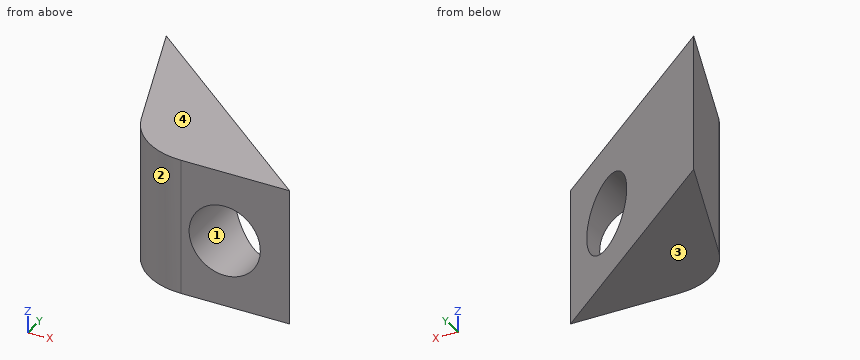
from build123d import *

# Parameters (mm, degrees)
BOSS_EXTRUDE1_DEPTH = 10
FILLET1_R           = 5
SKETCH4_R           = 2.6
CUT_EXTRUDE1_DEPTH  = 10


with BuildPart() as part:
    # Sketch2 → Boss-Extrude1 (new body)
    with BuildSketch(Plane.XY):
        Polygon((0, 0), (11.45, 0), (-4.62309301, 13.05), align=None)
    extrude(amount=BOSS_EXTRUDE1_DEPTH)

    # Fillet1
    fillet1_edges = [part.edges().sort_by_distance(p)[0] for p in [
        (0, 0, 5),
    ]]
    fillet(fillet1_edges, radius=FILLET1_R)

    # Sketch4 → Cut-Extrude1 (cut)
    with BuildSketch(Plane.XZ):
        with Locations(Location((6.713179585, 4.87, 0), (0, 0, 270))):
            Circle(SKETCH4_R)
    extrude(amount=-CUT_EXTRUDE1_DEPTH, mode=Mode.SUBTRACT)


solid = part.part
Geometry: final body of the model. Coordinates: model frame, mm. Face numbers are marked on the shaded views. Coordinates: 2 decimals unless noted, no trailing zeros. Loops run counter-clockwise (first coordinate to the right, second up) from the corner with the lowest first, then second, coordinate; pieces in that order, holes last. Notation, with made-up numbers: M 19.5,16.5 L 75.5,16.5 A23 cw 75.5,31.5 Z; hole C 26.5,73.5 d10. An arc over 180 degrees is marked long. One line per item, written item: value. Start each with the question number.
1) Draft query along Z for the marked faces 1, 2, 3 and 4. Return one class per face: released by +Z, released by -Z, zero draft, split by the parting line, or undercut.
2) Cut plane B-B (z = 2.75). Return loops of the section in (x, y), then the cut area to 3 significant figures.
3) Cut plane A-A (x = 8). Return loops of the section in (y, z), then the cut area to 3 significant figures.
4) Cut plane C-C (y = 1.5). Return loops of the section in (x, z), then the cut area to 3 significant figures.
5) Material intervals for L1, parallel to Y at x = 2.25, z = 3.5; L2, parallel to Y at x = 5, z = 1.75; L3, parallel to X at y = 9, z = 4, sorted ascending. Write a range as from..to.
6) Pin query (flat end, axial travel): P1, Ø5, axis at y = 7.5, z = 7, coming from the +X side; P2, Ø1.5, axis at x = -1, y = 9.5, coming from the -Z side; P3, Ø1.5, axis at y = 11.5, z = 3.5, coming from the -X side. Return the tip coordinate at first contact, or that it passes through.
7) Cut plane D-D (y = 3). Return loops of the section in (x, z), then the cut area to 3 significant figures.
Evaluation:
1. face 1: undercut
1. face 2: zero draft
1. face 3: released by -Z
1. face 4: released by +Z
2. outline: M -4.62,13.05 L -1.18,3.33 A5 ccw 3.53,0 L 5.21,0 L 5.21,5.07 Z; M 8.22,0 L 11.45,0 L 8.22,2.62 Z
2. area: 60.8 mm^2
3. outline: M 0,0 L 2.8,0 L 2.8,2.61 L 0,2.61 Z; M 0,7.13 L 2.8,7.13 L 2.8,10 L 0,10 Z
3. area: 15.4 mm^2
4. outline: M -0.04,0 L 9.6,0 L 9.6,10 L -0.04,10 Z; hole C 6.71,4.87 d5.2
4. area: 75.2 mm^2
5. L1: 0.17..7.47
5. L2: 0..5.24
5. L3: -3.19..0.37
6. P1: x = 5.29
6. P2: z = 0
6. P3: x = -4.34
7. outline: M -1.05,0 L 7.76,0 L 7.76,2.49 A2.6 cw long 7.76,7.25 L 7.76,10 L -1.05,10 Z
7. area: 72.2 mm^2
